Autodesk Inventor part; units mm, degrees
ref_plane "YZ Plane" through (0, 0, 0) normal (1, 0, 0) x (0, 1, 0)
ref_plane "XZ Plane" through (0, 0, 0) normal (0, 1, 0) x (-1, 0, 0)
ref_plane "XY Plane" through (0, 0, 0) normal (0, 0, 1) x (1, 0, 0)
sketch "Sketch1" plane through (0, 0, 0) normal (0, 0, 1) x (1, 0, 0)
  line L0 (-3.5, 27) -> (-3.5, 11.55)
  line L1 (-3.5, 11.55) -> (-2.45, 10.5)
  line L2 (-2.45, 10.5) -> (-2.45, 0)
  line L3 (-2.45, 0) -> (0, 0)
  line L4 (0, 27) -> (0, 0) construction
  line L5 (-3, 27) -> (-2.1, 25.4412)
  line L6 (-2.1, 25.4412) -> (-2.1, 0)
  line L7 (-3, 27) -> (-3.5, 27)
  dimension "d1" = 10.5
  dimension "d2" = 2.45
  dimension "d3" = 3.5
  dimension "d4" = 30
  dimension "d5" = 2.1
  dimension "d6" = 135
  dimension "d7" = 0.5
  dimension "d8" = 27
revolve "Revolution1" add sketch "Sketch1" angle 360 about axis through (0, 27, 0) along (0, -1, 0)
properties part number "ENDER 3 HEATBREAK" material "Aluminum 6061, Welded"
Here's how the part is built. I have some questions about the finished solid (model axes, mm). Give positions to 0.01 mm unless a question says otherwise; leave off trailing zeros. Loops run counter-clockwise (first coordinate to the right, second up) from the corner with the lowest first, then second, coordinate; pieces in that order, holes last. Notation, with made-up numbers: M 22.5,32.25 L 67.5,32.25 A13 ccw 67.5,50.25 Z; hole C -18.75,-8 d9. An arc over 180 degrees is marked long. Return JSON: item names as keys, results as strings.
Item 1: Imagine slicing it at D-D on y = 9.75. List the corners of the cut face in (x, z) for me.
A:
{"outline": "C 0,0 d4.9; hole C 0,0 d4.2"}
Item 2: I'm going to push a flat-ended pin straight in: pin 1 Ø3 at (x, z) = (-0.5, -1.5) entering from -Y. Where does the tip first touch, or does it pass through?
A:
{"pin 1": "stops at y = 0"}
Item 3: Thinking about a two-plate mould opening in Z: for faces 1 (the cylindrical face through (0.5, 5.2, 2.4)), 2 (the cylindrical face through (-2.003, 12.543, -0.631)), 3 (the flat face through (-3, 27, -1)), which applies, released by +Z, released by -Z, zero draft, split by the parting line, or undercut?
A:
{"face 1": "split by the parting line", "face 2": "undercut", "face 3": "zero draft"}
Item 4: Imagine slicing it at B-B on x = 0. List the corners of the cut face in (y, z) for me, then the cut area to 3 significant figures.
A:
{"outline": "M 0,-2.45 L 10.5,-2.45 L 11.55,-3.5 L 27,-3.5 L 27,-3 L 25.44,-2.1 L 0,-2.1 Z; M 0,2.1 L 25.44,2.1 L 27,3 L 27,3.5 L 11.55,3.5 L 10.5,2.45 L 0,2.45 Z", "area": "51.0 mm^2"}
Item 5: Imagine slicing it at C-C on y = 12.5. List the corners of the cut face in (x, z) for me.
A:
{"outline": "C 0,0 d7; hole C 0,0 d4.2"}
Item 6: Please list where these lines run through material, in increasing order: line 1 (X direction, y = 13, z = 0); line 2 (X direction, y = 5.25, z = 0).
A:
{"line 1": "x = -3.5 to -2.1, 2.1 to 3.5", "line 2": "x = -2.45 to -2.1, 2.1 to 2.45"}
Item 7: Imagine slicing it at A-A on z = 0. List the corners of the cut face in (x, y) for me, then the cut area to 3 significant figures.
A:
{"outline": "M -3.5,11.55 L -2.45,10.5 L -2.45,0 L -2.1,0 L -2.1,25.44 L -3,27 L -3.5,27 Z; M 2.1,0 L 2.45,0 L 2.45,10.5 L 3.5,11.55 L 3.5,27 L 3,27 L 2.1,25.44 Z", "area": "51.0 mm^2"}
